Autodesk Inventor part; units mm, degrees
ref_plane "YZ Plane" through (0, 0, 0) normal (1, 0, 0) x (0, 1, 0)
ref_plane "XZ Plane" through (0, 0, 0) normal (0, 1, 0) x (-1, 0, 0)
ref_plane "XY Plane" through (0, 0, 0) normal (0, 0, 1) x (1, 0, 0)
sketch "스케치1" plane through (0, 0, 0) normal (0, 0, 1) x (1, 0, 0)
  line L0 (-48.1, 15) -> (48.1, 15)
  line L1 (48.1, 15) -> (48.1, -15)
  line L2 (48.1, -15) -> (-48.1, -15)
  line L3 (-48.1, -15) -> (-48.1, 15)
  line L4 (-48.1, 15) -> (48.1, -15) construction
  line L5 (48.1, 15) -> (-48.1, -15) construction
  point P0 (0, 0)
  dimension "d0" = 96.2
  dimension "d1" = 30
extrude "돌출1" add sketch "스케치1" along normal blind 4
sketch "스케치2" plane through (0, 0, 4) normal (0, 0, 1) x (1, 0, 0)
  circle A0 centre (42.1, 0) radius 4.25
  circle A1 centre (-42.1, 0) radius 4.25
  arc A2 (-46.1, 15) -> (-48.1, 13) centre (-46.1, 13) ccw
  line L0 (-48.1, 13) -> (-48.1, -13)
  arc A3 (-48.1, -13) -> (-46.1, -15) centre (-46.1, -13) ccw
  line L1 (-46.1, -15) -> (46.1, -15)
  arc A4 (46.1, -15) -> (48.1, -13) centre (46.1, -13) ccw
  line L2 (48.1, -13) -> (48.1, 13)
  arc A5 (48.1, 13) -> (46.1, 15) centre (46.1, 13) ccw
  line L3 (46.1, 15) -> (-46.1, 15)
  circle A6 centre (12, 0) radius 1.35
  circle A7 centre (0, 12) radius 1.35
  circle A8 centre (-12, 0) radius 1.35
  circle A9 centre (42.1, -12) radius 1.8
  circle A10 centre (-42.1, -12) radius 1.8
  circle A11 centre (42.1, 12) radius 1.8
  circle A12 centre (-42.1, 12) radius 1.8
  line L4 (-48.1, -15) -> (48.1, -15)
  line L5 (48.1, -15) -> (48.1, 15)
  line L6 (48.1, 15) -> (-48.1, 15)
  line L7 (-48.1, 15) -> (-48.1, -15)
  point P0 (0, 0)
  point P1 (0, 0)
  point P2 (48.1, -13)
  point P3 (-48.1, 13)
  dimension "d4" = 8.5
  dimension "d5" = 92.2
  dimension "d6" = 26
  dimension "d7" = 8.5
  dimension "d8" = 15
  dimension "d9" = 15
  dimension "d10" = 6
  dimension "d11" = 6
  dimension "d12" = 12
  dimension "d13" = 12
  dimension "d14" = 3.6
  dimension "d15" = 3.6
  dimension "d16" = 3.6
  dimension "d17" = 3.6
  dimension "d18" = 12
  dimension "d19" = 12
  dimension "d20" = 2.7
  dimension "d21" = 2.7
  dimension "d22" = 2.7
  dimension "d25" = 12
  dimension "d26" = 24
extrude "돌출2" cut sketch "스케치2" against normal blind 4 contours A0 | A1 | A2 L7 L6 | L6 L5 A5 | A3 L4 L7 | L5 L4 A4 | A6 | A7 | A8 | A9 | A10 | A11 | A12
sketch "스케치3" plane through (0, 0, 4) normal (0, 0, 1) x (1, 0, 0)
  circle A0 centre (-12, 0) radius 1.35
  circle A1 centre (42.1, 0) radius 4.25
  circle A2 centre (-42.1, -12) radius 1.8
  circle A3 centre (42.1, 12) radius 1.8
  circle A4 centre (0, 12) radius 1.35
  circle A5 centre (-42.1, 0) radius 4.25
  circle A6 centre (-42.1, 12) radius 1.8
  circle A7 centre (42.1, -12) radius 1.8
  circle A8 centre (12, 0) radius 1.35
  arc A9 (46.1, -15) -> (48.1, -13) centre (46.1, -13) ccw
  line L0 (48.1, -13) -> (48.1, 13)
  arc A10 (48.1, 13) -> (46.1, 15) centre (46.1, 13) ccw
  line L1 (46.1, 15) -> (-46.1, 15)
  arc A11 (-46.1, 15) -> (-48.1, 13) centre (-46.1, 13) ccw
  line L2 (-48.1, 13) -> (-48.1, -13)
  arc A12 (-48.1, -13) -> (-46.1, -15) centre (-46.1, -13) ccw
  line L3 (-46.1, -15) -> (46.1, -15)
  line L4 (-48.1, 13) -> (-48.1, -13)
  line L5 (-48.1, 13) -> (-48.1, 16)
  arc A13 (48.1, 13) -> (46.1, 15) centre (46.1, 13) ccw
  line L6 (48.1, 13) -> (48.1, 16)
  line L7 (48.1, 16) -> (-48.1, 16)
  line L8 (48.1, -13) -> (48.1, 13)
  line L9 (48.1, -13) -> (48.1, -16)
  line L10 (-48.1, -13) -> (-48.1, -16)
  line L11 (-48.1, -16) -> (48.1, -16)
  point P0 (0, 0)
  dimension "d29" = 3
  dimension "d30" = 3
  dimension "d31" = 3
  dimension "d32" = 3
extrude "돌출3" add sketch "스케치3" against normal blind 4 contours A9 L9 L11 L10 A12 L3 | A10 L1 A11 L5 L7 L6
fillet "모깎기1" radius 3 4 edges at (-48.1, -16, 2) (48.1, -16, 2) (48.1, 16, 2) (-48.1, 16, 2)
sketch "스케치4" plane through (0, 0, 4) normal (0, 0, 1) x (1, 0, 0)
  arc A0 (-45.1, 16) -> (-48.1, 13) centre (-45.1, 13) ccw
  line L0 (-48.1, 13) -> (-48.1, -13)
  arc A1 (-48.1, -13) -> (-45.1, -16) centre (-45.1, -13) ccw
  line L1 (-45.1, -16) -> (45.1, -16)
  arc A2 (45.1, -16) -> (48.1, -13) centre (45.1, -13) ccw
  line L2 (48.1, -13) -> (48.1, 13)
  arc A3 (48.1, 13) -> (45.1, 16) centre (45.1, 13) ccw
  line L3 (45.1, 16) -> (-45.1, 16)
  circle A4 centre (-12, 0) radius 1.35
  circle A5 centre (42.1, 0) radius 4.25
  circle A6 centre (-42.1, -12) radius 1.8
  circle A7 centre (42.1, 12) radius 1.8
  circle A8 centre (0, 12) radius 1.35
  circle A9 centre (-42.1, 0) radius 4.25
  circle A10 centre (-42.1, 12) radius 1.8
  circle A11 centre (42.1, -12) radius 1.8
  circle A12 centre (12, 0) radius 1.35
  line L4 (45.1, 16) -> (-45.1, 16)
  line L5 (-45.1, 16) -> (-51.1, 16)
  arc A13 (-45.1, 16) -> (-48.1, 13) centre (-45.1, 13) ccw
  line L6 (-51.1, 16) -> (-51.1, -16)
  line L7 (-45.1, -16) -> (45.1, -16)
  line L8 (-51.1, -16) -> (-45.1, -16)
  line L9 (45.1, 16) -> (51.1, 16)
  line L10 (51.1, 16) -> (51.1, -16)
  line L11 (51.1, -16) -> (45.1, -16)
  point P0 (0, 0)
  dimension "d36" = 6
  dimension "d37" = 6
extrude "돌출4" add sketch "스케치4" against normal blind 4 contours A0 L0 A1 L8 L6 L5 | L9 L10 L11 A2 L2 A3
fillet "모깎기2" radius 3 4 edges at (-51.1, -16, 2) (-51.1, 16, 2) (51.1, 16, 2) (51.1, -16, 2)
sketch "스케치5" plane through (0, 0, 4) normal (0, 0, 1) x (1, 0, 0)
  circle A0 centre (0, 0) radius 4.25
  dimension "d41" = 8.5
extrude "돌출5" cut sketch "스케치5" against normal blind 4
sketch "스케치6" plane through (0, 0, 4) normal (0, 0, 1) x (1, 0, 0)
  line L0 (0, 0) -> (0, 10)
  circle A0 centre (0, 0) radius 4.25
  line L1 (0, 0) -> (0, -10)
  circle A1 centre (0, 10) radius 1.8
  circle A2 centre (0, -10) radius 1.8
  circle A3 centre (0, 0) radius 4.25
  arc A4 (48.1, -16) -> (51.1, -13) centre (48.1, -13) ccw
  line L2 (51.1, -13) -> (51.1, 13)
  arc A5 (51.1, 13) -> (48.1, 16) centre (48.1, 13) ccw
  line L3 (48.1, 16) -> (-48.1, 16)
  arc A6 (-48.1, 16) -> (-51.1, 13) centre (-48.1, 13) ccw
  line L4 (-51.1, 13) -> (-51.1, -13)
  arc A7 (-51.1, -13) -> (-48.1, -16) centre (-48.1, -13) ccw
  line L5 (-48.1, -16) -> (48.1, -16)
  circle A8 centre (-12, 0) radius 1.35
  circle A9 centre (42.1, 0) radius 4.25
  circle A10 centre (-42.1, -12) radius 1.8
  circle A11 centre (42.1, 12) radius 1.8
  circle A12 centre (0, 12) radius 1.35
  circle A13 centre (-42.1, 0) radius 4.25
  circle A14 centre (-42.1, 12) radius 1.8
  circle A15 centre (42.1, -12) radius 1.8
  circle A16 centre (12, 0) radius 1.35
  dimension "d44" = 10
  dimension "d45" = 10
  dimension "d46" = 3.6
  dimension "d47" = 3.6
extrude "돌출6" add sketch "스케치6" against normal blind 4 contours A12 A1 | A1 A12 | A8 | A16 picked at (0.3966, 12.2209) picked at (0.1959, 11.4027)
extrude "돌출7" cut sketch "스케치6" against normal blind 4 contours A1 A12 | A2 | A1 A12 picked at (-0.1974, 9.0374) picked at (0.1959, 11.4027)
sketch "스케치8" plane through (-48.1, -16, 4) normal (0, -1, 0) x (1, 0, 0)
  line L0 (96.2, 0) -> (96.2, -4)
  line L1 (0, 0) -> (96.2, 0)
  line L2 (0, -4) -> (0, 0)
  line L3 (96.2, -4) -> (0, -4)
  line L4 (96.2, -4) -> (96.2, 0)
  line L5 (96.2, -2) -> (0, -2) construction
  line L6 (0, -4) -> (0, 0)
  line L7 (48.1, -4) -> (48.1, 0) construction
  circle A0 centre (34.1, -2) radius 1.25
  circle A1 centre (24.1, -2) radius 1.25
  circle A2 centre (14.1, -2) radius 1.25
  circle A3 centre (62.1, -2) radius 1.25
  circle A4 centre (72.1, -2) radius 1.25
  circle A5 centre (82.1, -2) radius 1.25
  point P0 (48.1, -2)
  dimension "d53" = 2.5
  dimension "d54" = 2.5
  dimension "d55" = 2.5
  dimension "d56" = 2.5
  dimension "d57" = 2.5
  dimension "d58" = 2.5
  dimension "d59" = 14
  dimension "d60" = 10
  dimension "d61" = 10
  dimension "d63" = 10
  dimension "d64" = 10
  dimension "d67" = 14
extrude "돌출8" cut sketch "스케치8" against normal blind 4 contours A0 | A1 | A2 | A3 | A4 | A5
mirror "미러1" about plane through (0, 0, 0) normal (0, 1, 0) of "돌출8"
properties part number "스프링블럭2" material "알루미늄 6061"
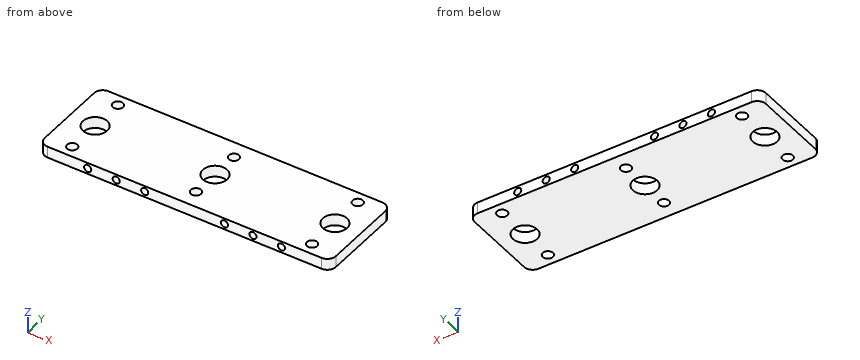
Source: CAD feature listing. Evaluate the final solid. Frame: model axes, mm. Round coordinates to 2 decimals unless told otherwise and drop trailing zeros. Loops run counter-clockwise (first coordinate to the right, second up) from the corner with the lowest first, then second, coordinate; pieces in that order, holes last. Notation, with made-up numbers: M 51,39 L 65,39 A22 ccw 65,50 Z; hole C -6,54.5 d5. An arc over 180 degrees is marked long. Return JSON: item names as keys, results as strings. Group by question number.
1. Section query B-B on y = 2. Output: boundary loops of the cut face in (x, z), and give its area (3 significant figures).
2. Section query D-D on z = 2. State how many separate pieces and enclosed holes the cut face has, and give its area (3 significant figures).
3. Section query A-A on x = 0. Output: boundary loops of the cut face in (y, z).
4. Section query C-C on x = 14. Output: boundary loops of the cut face in (y, z), and give its area (3 significant figures).
5. Material intervals for line 1 along Y through (x, z) = (42.1, 0.95); line 2 along Z through (x, y) = (34, 14.1); line 3 along X through (y, z) = (10.5, 2.15), sorted ascending. Write a range as from..to.
6. Pin query (flat end, axial travel): pin 1 (2 mm diameter, centred on x = -34, z = 2, fed in from -Y); pin 2 (1.2 mm diameter, centred on x = 14.5, z = 2, fed in from +Y); pin 3 (2 mm diameter, centred on x = 32, y = -4.5, fed in from -Z). Return the tip coordinate at first contact, or that it passes through.
Checks:
{
 "1": {"outline": "M -51.1,0 L -45.85,0 L -45.85,4 L -51.1,4 Z; M -38.35,0 L -3.75,0 L -3.75,4 L -38.35,4 Z; M 3.75,0 L 38.35,0 L 38.35,4 L 3.75,4 Z; M 45.85,0 L 51.1,0 L 51.1,4 L 45.85,4 Z", "area": "319 mm²"},
 "2": {"separate pieces": "1", "enclosed holes": "9", "area": "2,910 mm²"},
 "3": {"outline": "M -16,0 L -11.8,0 L -11.8,4 L -16,4 Z; M -8.2,0 L -4.25,0 L -4.25,4 L -8.2,4 Z; M 4.25,0 L 8.2,0 L 8.2,4 L 4.25,4 Z; M 11.8,0 L 16,0 L 16,4 L 11.8,4 Z"},
 "4": {"outline": "M -16,0 L 16,0 L 16,0.75 L 12,0.75 L 12,3.25 L 16,3.25 L 16,4 L -16,4 L -16,3.25 L -12,3.25 L -12,0.75 L -16,0.75 Z", "area": "108 mm²"},
 "5": {"line 1": "y = -16..-13.8, -10.2..-4.25, 4.25..10.2, 13.8..16", "line 2": "z = 0..0.75, 3.25..4", "line 3": "x = -51.1..-43.09, -41.11..-1.73, 1.73..41.11, 43.09..51.1"},
 "6": {"pin 1": "stops at y = -12", "pin 2": "stops at y = 12", "pin 3": "stops at z = 0"}
}
